from build123d import *

# Parameters (mm, degrees)
F0_W     = 5
F0_H     = 9.9937266076
F1_DEPTH = 20
F2_DEPTH = 158.6
F5_D     = 3
F5_DEPTH = 5
F5_TIP   = 0.9012909285
F6_D     = 3
F6_DEPTH = 5
F6_TIP   = 0.9012909285


with BuildPart() as f1:
    # F0 (on Top) → F1 (new body)
    with BuildSketch(Plane.XY):
        Polygon((17.5, 18.631580086), (-22.5, 18.631580086), (-22.5, -7.8947371674), (-5, -7.8947371674), (-5, 2.0989894401), (-5, 2.1052628326), (0, 2.1052628326), (0, 2.0989894401), (0, -7.8947371674), (17.5, -7.8947371674), align=None)
        with Locations((-2.5, -2.8978738637)):
            Rectangle(F0_W, F0_H)
    extrude(amount=F1_DEPTH)

    # F0 (on Top) → F2 (cut)
    with BuildSketch(Plane.XY):
        with Locations((-2.5, -2.8978738637)):
            Rectangle(F0_W, F0_H)
    extrude(amount=F2_DEPTH, mode=Mode.SUBTRACT)

    # F5
    with Locations(Plane(origin=(-22.5, 0, 0), x_dir=(0, -1, 0), z_dir=(-1, 0, 0))):
        with Locations((-5.3684214593, 10)):
            Hole(F5_D / 2, depth=F5_DEPTH)
            with Locations((0, 0, -(F5_DEPTH + F5_TIP / 2))):  # 118° drill point
                Cone(0, F5_D / 2, F5_TIP, mode=Mode.SUBTRACT)

    # F6
    with Locations(Plane.YZ.offset(17.5)):
        with Locations((5.357359536, 10.0329257548)):
            Hole(F6_D / 2, depth=F6_DEPTH)
            with Locations((0, 0, -(F6_DEPTH + F6_TIP / 2))):  # 118° drill point
                Cone(0, F6_D / 2, F6_TIP, mode=Mode.SUBTRACT)


solid = f1.part
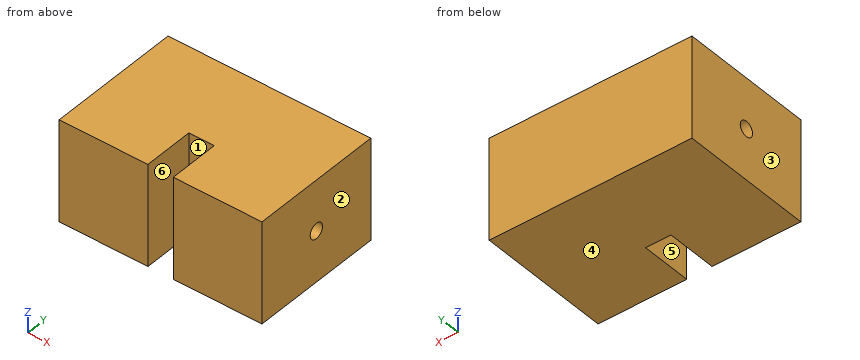
Verification items for the finished model (mm, model axes). Face numbers are marked on the shaded views. A direction names the side the tool comes from. Round coordinates to 2 decimals unless told otherwise and drop trailing zeros. Loops run counter-clockwise (first coordinate to the right, second up) from the corner with the lowest first, then second, coordinate; pieces in that order, holes last. Notation, with made-up numbers: (81, 19.25) - (136, 19.25) arc R22 cw to (136, 44.25) - close; hole circle Ø3 at (-5, -6). An arc over 180 degrees is marked (long way). Answer in a Markdown table with one row per item. Add a question column.
Q1. Tool access check on the marked faces 1 and 2. Record the directions out of +Z, -Z, +X, -X, +Y, -Y that give a thin tool (end or side, any length) a straight path to the whole face; none if there is none.
Q2. Section check B-B on z = 5.5. Enter the section's corners in (x, y).
Q3. Release check for a two-part mould opening along X. For the marked faces 3, 4, 5 and 6 record: pulls with the +X half, pulls with the -X half, needs draft (parallel to the pull), parting line crosses it, or undercut.
Q4. Gauge pin test, flat end, axial feed: pin 1 (2.5 mm diameter, centred on y = 5.36, z = 10.03, fed in from -X). Record the tip position at first contact, or that the pin passes through.
Q5. Section check A-A on y = -2.5. Enter the section's corners in (x, z), plus the area to 3 significant figures.
Q6. Material ranges on line 1 (X direction, y = -2, z = 7); line 2 (Y direction, x = -19.05, z = 10); line 3 (Y direction, x = -1, z = 8.25), recorded low to high.
Found:
| question | item | result |
|---|---|---|
| 1 | face 1 | +Z, -Z, -Y |
| 1 | face 2 | +Z, -Z, +X, +Y, -Y |
| 2 | outline | (-22.5, -7.89) - (-5, -7.89) - (-5, 2.11) - (0, 2.11) - (0, -7.89) - (17.5, -7.89) - (17.5, 18.63) - (-22.5, 18.63) - close |
| 3 | face 3 | pulls with the -X half |
| 3 | face 4 | needs draft |
| 3 | face 5 | undercut |
| 3 | face 6 | undercut |
| 4 | pin 1 | stops at x = -17.37 |
| 5 | outline | (-22.5, 0) - (-5, 0) - (-5, 20) - (-22.5, 20) - close; (0, 0) - (17.5, 0) - (17.5, 20) - (0, 20) - close |
| 5 | area | 700 mm² |
| 6 | line 1 | x = -22.5 to -5, 0 to 17.5 |
| 6 | line 2 | y = -7.89 to 3.87, 6.87 to 18.63 |
| 6 | line 3 | y = 2.11 to 18.63 |
